The drawing under review shows one solid part. Ordinate dimensions are in mm from its lowest x, y, z. Give positions to 0.01 mm unless a question says otherwise; leave off trailing zeros. Order: outer loops, then holes, each group sorted by start corner. A loop starts at its lowest first (then second) coordinate and runs counter-clockwise, first axis right, second up. Notation, with made-up numbers: (62.25, 89.25) -> (113.25, 89.25) arc R23 cw to (113.25, 123.25) -> close; hole circle Ø3 at (6.25, 70). An arc over 180 degrees is marked (long way). Use CSV: the item, a comma, the result in double quotes. Start each with the question number.
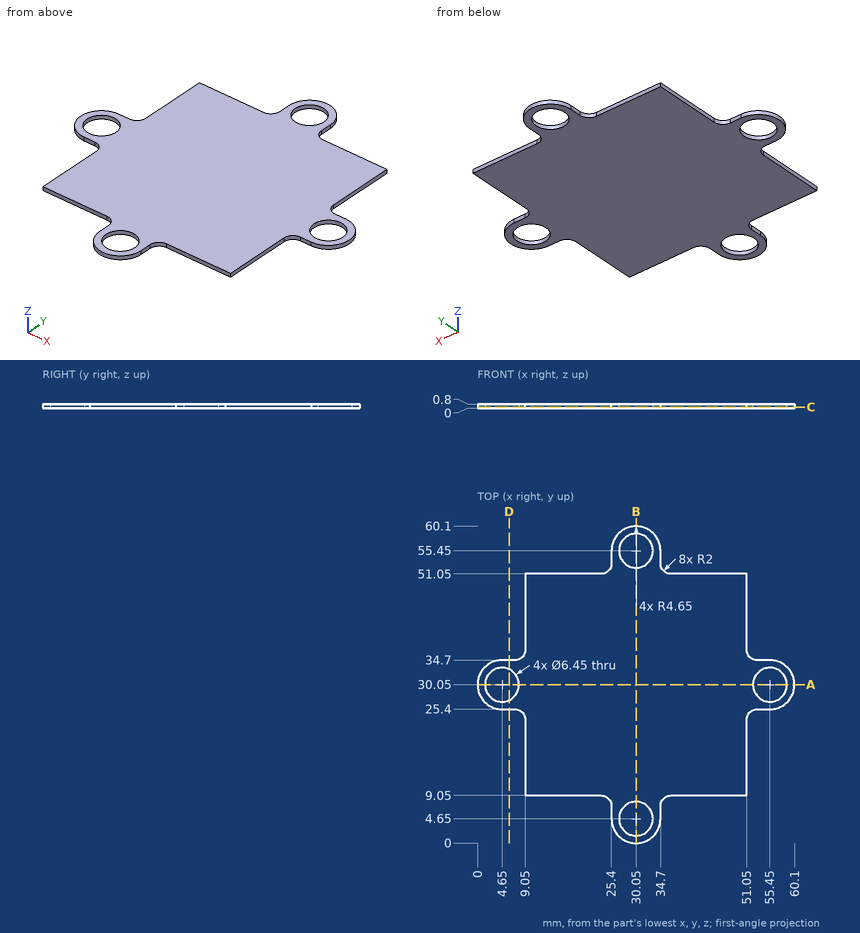
1. Consider section C-C (z = 0.2). State how many separate pieces and enclosed holes the cut face has, plus the area to 3 significant figures.
2. Consider section D-D (x = 6). State the section outline as (y, z) points, plus the area to 3 significant figures.
3. To check wall thickness, follow L1, parallel to Y at x = 30.05, z = 0.4 (3 decimals); L2, parallel to Y at x = 55.45, z = 0.45 (3 decimals); L3, parallel to X at y = 27.5, z = 0.4. State the ranges of each line that lie inside material, in increasing order. Write a range as [from, to].
4. Consider section A-A (y = 30.05). State the section outline as (x, z) points (3 decimals), plus the area to 3 significant figures.
Answer list:
1,separate pieces,"1"
1,enclosed holes,"4"
1,area,"1,940 mm2"
2,outline,"(25.4, 0) -> (27.12, 0) -> (27.12, 0.8) -> (25.4, 0.8) -> close; (32.98, 0) -> (34.7, 0) -> (34.7, 0.8) -> (32.98, 0.8) -> close"
2,area,"2.75 mm2"
3,L1,"[0, 1.425], [7.875, 52.225], [58.675, 60.1]"
3,L2,"[25.4, 26.825], [33.275, 34.7]"
3,L3,"[0.76, 2.68], [6.62, 53.48], [57.42, 59.34]"
4,outline,"(0, 0) -> (1.425, 0) -> (1.425, 0.8) -> (0, 0.8) -> close; (7.875, 0) -> (52.225, 0) -> (52.225, 0.8) -> (7.875, 0.8) -> close; (58.675, 0) -> (60.1, 0) -> (60.1, 0.8) -> (58.675, 0.8) -> close"
4,area,"37.8 mm2"
